Geometry check sheet. Reference: the model listing, model coordinates, mm. A direction names the side the tool comes from. Coordinates: 2 decimals unless noted, no trailing zeros. Write each loop counter-clockwise with the first axis right and the second up, starting at its lowest first coordinate (ties: lowest second). Pieces come first, ordered by that corner, then holes. Notation, with made-up numbers: (6.5, -22) -> (43.5, -22) arc R16 cw to (43.5, -14) -> close; hole circle Ø11 at (-29.75, 0.5). An arc over 180 degrees is marked (long way). Answer in a Markdown table with one row per item. Add a question column.
Q1. Section check C-C, the plane y = 1.6. Count the separate pieces of the cut face and the enclosed holes in it, and give its area (3 significant figures).
Q2. Section check A-A, the plane x = -55. Record the boundary of the cut face in (y, z), and give its area (3 significant figures).
Q3. Tool access check on faces 5 (the face through (9, 2, -46)), 6 (the face through (-2, 0, -1)). Record the directions out of +Z, -Z, +X, -X, +Y, -Y that give a thin tool (end or side, any length) a straight path to the whole face; none if there is none.
Q4. Release check for a two-part mould opening along X. For faces 1 (the face through (-2, 3, -1)), 2 (the face through (-107.15, 1.48, 58.99)), 3 (the face through (-99, 2, -46)), 4 (the face through (106.99, 1.48, 59.15)) record: pulls with the +X half, pulls with the -X half, needs draft (parallel to the pull), parting line crosses it, or undercut.
Q5. Section check B-B, the plane x = 55. Record the boundary of the cut face in (y, z), and give its area (3 significant figures).
Q6. Gauge pin test, flat end, axial feed: P1, Ø0.9, axis at y = 1.5, z = 54.5, coming from the -X side. Record the tip position at first contact, or that the pin passes through.
Q7. Thickness scan on line 1 (Z direction, x = -47.5, y = 0.4); line 2 (Z direction, x = -90, y = 1.95); line 3 (Z direction, x = 87, y = 0.6). Record the ranges inside material, lowest first.
```python
from build123d import *

# Parameters (mm, degrees)
SKETCH1_R           = 1.35
BOSS_EXTRUDE1_DEPTH = 3
SKETCH4_R           = 1.5
SKETCH4_W           = 40
SKETCH4_H           = 3
CUT_EXTRUDE1_DEPTH  = 3
SKETCH5_R           = 1.7
SKETCH5_R_2         = 1.75
CUT_EXTRUDE2_DEPTH  = 3
SKETCH6_R           = 0.5
CUT_EXTRUDE3_DEPTH  = 3
SKETCH7_R           = 1.5
CUT_EXTRUDE4_DEPTH  = 3
CUT_EXTRUDE5_DEPTH  = 3
SKETCH9_W           = 15
SKETCH9_H           = 3
CUT_EXTRUDE6_DEPTH  = 3


with BuildPart() as part:
    # Sketch1 → Boss-Extrude1 (new body)
    with BuildSketch(Plane(origin=(0, 0, 0), x_dir=(1, 0, 0), z_dir=(0, 1, 0))):
        with BuildLine():
            Line((-100, -62), (100, -62))
            ThreePointArc((100, -62), (107.071067812, -59.071067812), (110, -52))
            Line((110, -52), (110, 52))
            ThreePointArc((110, 52), (107.071067812, 59.071067812), (100, 62))
            Line((100, 62), (-100, 62))
            ThreePointArc((-100, 62), (-107.071067812, 59.071067812), (-110, 52))
            Line((-110, 52), (-110, -52))
            ThreePointArc((-110, -52), (-107.071067812, -59.071067812), (-100, -62))
        make_face()
        with Locations(Location((69.472640088, 10.571681526, 0), (0, 0, 270))):
            Circle(SKETCH1_R, mode=Mode.SUBTRACT)
        with Locations(Location((11.472640088, -38.428318474, 0), (0, 0, 270))):
            Circle(SKETCH1_R, mode=Mode.SUBTRACT)
    extrude(amount=BOSS_EXTRUDE1_DEPTH)

    # Sketch4 → Cut-Extrude1 (cut)
    with BuildSketch(Plane(origin=(0, 3, 0), x_dir=(1, 0, 0), z_dir=(0, 1, 0))):
        with Locations(Location((0, -57.5, 0), (0, 0, 270))):
            Circle(SKETCH4_R)
        with Locations(Location((0, 57.5, 0), (0, 0, 90))):
            Circle(SKETCH4_R)
        with Locations((-40, -57.5)):
            Rectangle(SKETCH4_W, SKETCH4_H)
        with Locations((40, -57.5)):
            Rectangle(SKETCH4_W, SKETCH4_H)
        with Locations((-40, 57.5)):
            Rectangle(SKETCH4_W, SKETCH4_H)
        with Locations((40, 57.5)):
            Rectangle(SKETCH4_W, SKETCH4_H)
    extrude(amount=-CUT_EXTRUDE1_DEPTH, mode=Mode.SUBTRACT)

    # Sketch5 → Cut-Extrude2 (cut)
    with BuildSketch(Plane(origin=(0, 3, 0), x_dir=(1, 0, 0), z_dir=(0, 1, 0))):
        with Locations(Location((-95.681755145, 29.511348179, 0), (0, 0, 270))):
            Circle(SKETCH5_R)
        with Locations(Location((-95.425501916, -29.52854371, 0), (0, 0, 270))):
            Circle(SKETCH5_R_2)
        with Locations(Location((-6.575715248, -29.029034924, 0), (0, 0, 270))):
            Circle(SKETCH5_R_2)
        with Locations(Location((-6.581697253, 29.400968192, 0), (0, 0, 270))):
            Circle(SKETCH5_R_2)
    extrude(amount=-CUT_EXTRUDE2_DEPTH, mode=Mode.SUBTRACT)

    # Sketch6 → Cut-Extrude3 (cut)
    with BuildSketch(Plane(origin=(0, 3, 0), x_dir=(1, 0, 0), z_dir=(0, 1, 0))):
        with Locations(Location((32.222640088, -4.428318474, 0), (0, 0, 270))):
            Circle(SKETCH6_R)
        with Locations(Location((34.722640088, -4.428318474, 0), (0, 0, 270))):
            Circle(SKETCH6_R)
        with Locations(Location((37.222640088, -4.428318474, 0), (0, 0, 270))):
            Circle(SKETCH6_R)
        with Locations(Location((39.722640088, -4.428318474, 0), (0, 0, 270))):
            Circle(SKETCH6_R)
        with Locations((-29.984615318, 187.322240446)):
            Circle(SKETCH6_R)
        with Locations(Location((42.222640088, -4.428318474, 0), (0, 0, 270))):
            Circle(SKETCH6_R)
        with Locations(Location((32.222640088, -6.928318474, 0), (0, 0, 270))):
            Circle(SKETCH6_R)
        with Locations(Location((34.722640088, -6.928318474, 0), (0, 0, 270))):
            Circle(SKETCH6_R)
        with Locations(Location((37.222640088, -6.928318474, 0), (0, 0, 270))):
            Circle(SKETCH6_R)
        with Locations(Location((39.722640088, -6.928318474, 0), (0, 0, 270))):
            Circle(SKETCH6_R)
        with Locations(Location((42.222640088, -6.928318474, 0), (0, 0, 270))):
            Circle(SKETCH6_R)
        with Locations(Location((32.222640088, -9.428318474, 0), (0, 0, 270))):
            Circle(SKETCH6_R)
        with Locations(Location((34.722640088, -9.428318474, 0), (0, 0, 270))):
            Circle(SKETCH6_R)
        with Locations(Location((37.222640088, -9.428318474, 0), (0, 0, 270))):
            Circle(SKETCH6_R)
        with Locations(Location((39.722640088, -9.428318474, 0), (0, 0, 270))):
            Circle(SKETCH6_R)
        with Locations(Location((42.222640088, -9.428318474, 0), (0, 0, 270))):
            Circle(SKETCH6_R)
        with Locations(Location((32.222640088, -11.928318474, 0), (0, 0, 270))):
            Circle(SKETCH6_R)
        with Locations(Location((34.722640088, -11.928318474, 0), (0, 0, 270))):
            Circle(SKETCH6_R)
        with Locations(Location((37.222640088, -11.928318474, 0), (0, 0, 270))):
            Circle(SKETCH6_R)
        with Locations(Location((39.722640088, -11.928318474, 0), (0, 0, 270))):
            Circle(SKETCH6_R)
        with Locations(Location((42.222640088, -11.928318474, 0), (0, 0, 270))):
            Circle(SKETCH6_R)
        with Locations(Location((32.222640088, -14.428318474, 0), (0, 0, 270))):
            Circle(SKETCH6_R)
        with Locations(Location((34.722640088, -14.428318474, 0), (0, 0, 270))):
            Circle(SKETCH6_R)
        with Locations(Location((37.222640088, -14.428318474, 0), (0, 0, 270))):
            Circle(SKETCH6_R)
        with Locations(Location((39.722640088, -14.428318474, 0), (0, 0, 270))):
            Circle(SKETCH6_R)
        with Locations(Location((42.222640088, -14.428318474, 0), (0, 0, 270))):
            Circle(SKETCH6_R)
    extrude(amount=-CUT_EXTRUDE3_DEPTH, mode=Mode.SUBTRACT)

    # Sketch7 → Cut-Extrude4 (cut)
    with BuildSketch(Plane(origin=(0, 3, 0), x_dir=(1, 0, 0), z_dir=(0, 1, 0))):
        with Locations(Location((-106.437330196, 6.5, 0), (0, 0, 270))):
            Circle(SKETCH7_R)
        with Locations(Location((-106.437330196, -6.5, 0), (0, 0, 270))):
            Circle(SKETCH7_R)
    extrude(amount=-CUT_EXTRUDE4_DEPTH, mode=Mode.SUBTRACT)

    # Sketch8 → Cut-Extrude5 (cut)
    with BuildSketch(Plane(origin=(0, 3, 0), x_dir=(1, 0, 0), z_dir=(0, 1, 0))):
        with BuildLine():
            Line((-95, 50), (5, 50))
            ThreePointArc((5, 50), (9, 46), (5, 42))
            Line((5, 42), (-95, 42))
            ThreePointArc((-95, 42), (-99, 46), (-95, 50))
        make_face()
        with BuildLine():
            Line((-95, -42), (5, -42))
            ThreePointArc((5, -42), (9, -46), (5, -50))
            Line((5, -50), (-95, -50))
            ThreePointArc((-95, -50), (-99, -46), (-95, -42))
        make_face()
    extrude(amount=-CUT_EXTRUDE5_DEPTH, mode=Mode.SUBTRACT)

    # Sketch9 → Cut-Extrude6 (cut)
    with BuildSketch(Plane(origin=(0, 3, 0), x_dir=(1, 0, 0), z_dir=(0, 1, 0))):
        with Locations((-77.5, -54.5)):
            Rectangle(SKETCH9_W, SKETCH9_H)
        with Locations((-77.5, 54.5)):
            Rectangle(SKETCH9_W, SKETCH9_H)
        with Locations((92.5, 54.5)):
            Rectangle(SKETCH9_W, SKETCH9_H)
        with Locations((92.5, -54.5)):
            Rectangle(SKETCH9_W, SKETCH9_H)
    extrude(amount=-CUT_EXTRUDE6_DEPTH, mode=Mode.SUBTRACT)


solid = part.part
```
Calculated:
| question | item | result |
|---|---|---|
| 1 | separate pieces | 1 |
| 1 | enclosed holes | 45 |
| 1 | area | 24,700 mm² |
| 2 | outline | (0, -62) -> (3, -62) -> (3, -59) -> (0, -59) -> close; (0, -56) -> (3, -56) -> (3, -50) -> (0, -50) -> close; (0, -42) -> (3, -42) -> (3, 42) -> (0, 42) -> close; (0, 50) -> (3, 50) -> (3, 56) -> (0, 56) -> close; (0, 59) -> (3, 59) -> (3, 62) -> (0, 62) -> close |
| 2 | area | 306 mm² |
| 3 | face 5 | +Y, -Y |
| 3 | face 6 | +Z, -Z, +X, -X, -Y |
| 4 | face 1 | needs draft |
| 4 | face 2 | pulls with the -X half |
| 4 | face 3 | undercut |
| 4 | face 4 | pulls with the +X half |
| 5 | outline | (0, -62) -> (3, -62) -> (3, -59) -> (0, -59) -> close; (0, -56) -> (3, -56) -> (3, 56) -> (0, 56) -> close; (0, 59) -> (3, 59) -> (3, 62) -> (0, 62) -> close |
| 5 | area | 354 mm² |
| 6 | P1 | stops at x = -109.79 |
| 7 | line 1 | z = -62 to -59, -56 to -50, -42 to 42, 50 to 56, 59 to 62 |
| 7 | line 2 | z = -62 to -50, -42 to 42, 50 to 62 |
| 7 | line 3 | z = -62 to -56, -53 to 53, 56 to 62 |
